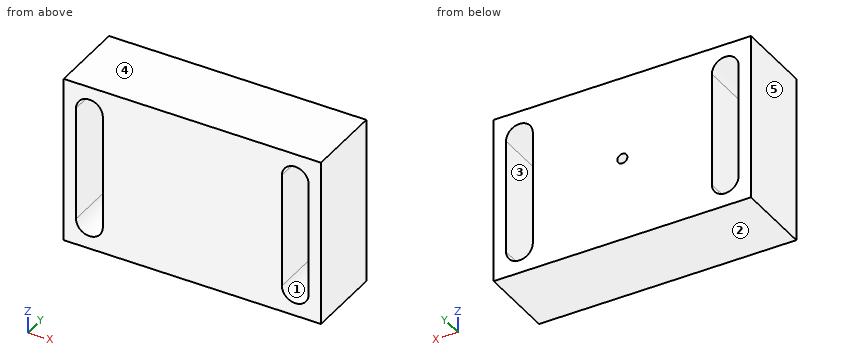
Autodesk Inventor part; units mm, degrees
ref_plane "YZ Plane" through (0, 0, 0) normal (1, 0, 0) x (0, 1, 0)
ref_plane "XZ Plane" through (0, 0, 0) normal (0, 1, 0) x (-1, 0, 0)
ref_plane "XY Plane" through (0, 0, 0) normal (0, 0, 1) x (1, 0, 0)
sketch "Sketch1" plane through (0, 0, 0) normal (0, 0, 1) x (1, 0, 0)
  line L0 (0, 0) -> (63.5, 0)
  line L1 (63.5, 0) -> (63.5, 19.05)
  line L2 (63.5, 19.05) -> (0, 19.05)
  line L3 (0, 19.05) -> (0, 0)
  dimension "d2" = 63.5
  dimension "d3" = 19.05
extrude "Extrusion1" add sketch "Sketch1" along normal blind 41.275
sketch "Sketch2" plane through (0, 19.05, 0) normal (0, 1, 0) x (1, 0, 0)
  line L0 (63.5, 0) -> (0, 0)
  line L1 (0, 0) -> (0, -41.275)
  point P0 (31.75, -20.6375)
  dimension "d4" = 20.6375
  dimension "d5" = 31.75
hole "Hole1" at (31.75, 19.05, 20.6375) direction (0, -1, 0) diameter 2.4638 depth 12.7 tip angle 118
sketch "Sketch3" plane through (0, 19.05, 0) normal (0, 1, 0) x (1, 0, 0)
  line L0 (6.35, -34.798) -> (6.35, -6.477) construction
  line L1 (3.048, -34.798) -> (3.048, -6.477)
  line L2 (9.652, -6.477) -> (9.652, -34.798)
  arc A0 (3.048, -34.798) -> (9.652, -34.798) centre (6.35, -34.798) ccw
  arc A1 (9.652, -6.477) -> (3.048, -6.477) centre (6.35, -6.477) ccw
  line L3 (0, 0) -> (0, -41.275)
  line L4 (63.5, -41.275) -> (0, -41.275)
  line L5 (63.5, 0) -> (0, 0)
  circle A2 centre (31.75, -20.6375) radius 1.2319
  circle A3 centre (31.75, -20.6375) radius 1.2319
  line L6 (31.75, -20.6375) -> (31.75, 0) construction
  line L7 (57.15, -34.798) -> (57.15, -6.477) construction
  line L8 (60.452, -34.798) -> (60.452, -6.477)
  line L9 (53.848, -6.477) -> (53.848, -34.798)
  arc A4 (53.848, -34.798) -> (60.452, -34.798) centre (57.15, -34.798) ccw
  arc A5 (60.452, -6.477) -> (53.848, -6.477) centre (57.15, -6.477) ccw
  point P0 (6.35, -20.6375)
  point P1 (57.15, -20.6375)
  dimension "d13" = 6.604
  dimension "d15" = 3.175
  dimension "d16" = 3.175
  dimension "d17" = 25.4
extrude "Extrusion2" cut sketch "Sketch3" against normal blind 25.4 contours L1 A1 L2 A0 | A4 L9 A5 L8
properties part number "Track Foot" material "Aluminum 6061"
For this review, take the finished solid that the model builds, in its own axes (mm). Face numbers are marked on the shaded views. A direction names the side the tool comes from. Round coordinates to 2 decimals unless told otherwise and drop trailing zeros. Write each loop counter-clockwise with the first axis right and the second up, starting at its lowest first coordinate (ties: lowest second). Pieces come first, ordered by that corner, then holes. Notation, with made-up numbers: (43.5, 0.25) -> (92.5, 0.25) arc R27 ccw to (92.5, 21.25) -> close; hole circle Ø5 at (-2.5, 27). An arc over 180 degrees is marked (long way). Use one line per item in the form item = value.
1) To check wall thickness, follow L1, parallel to X at y = 13.5, z = 35; L2, parallel to Z at x = 31.75, y = 12.25 (3 decimals). State the ranges of each line that lie inside material, in increasing order. Write a range as from..to.
Found:
L1 = 0..3.05, 9.65..53.85, 60.45..63.5
L2 = 0..19.406, 21.869..41.275
2) Take a section at A-A, the plane z = 11. Write out the cut boundary in (x, y).
Found:
outline = (0, 0) -> (3.05, 0) -> (3.05, 19.05) -> (0, 19.05) -> close; (9.65, 0) -> (53.85, 0) -> (53.85, 19.05) -> (9.65, 19.05) -> close; (60.45, 0) -> (63.5, 0) -> (63.5, 19.05) -> (60.45, 19.05) -> close
3) Take a section at D-D, the plane y = 3.75. Write out the cut boundary in (x, z) (3 decimals), and give its area (3 significant figures).
Found:
outline = (0, 0) -> (63.5, 0) -> (63.5, 41.275) -> (0, 41.275) -> close; hole (3.048, 6.477) arc R3.302 ccw to (9.652, 6.477) -> (9.652, 34.798) arc R3.302 ccw to (3.048, 34.798) -> close; hole (53.848, 6.477) arc R3.302 ccw to (60.452, 6.477) -> (60.452, 34.798) arc R3.302 ccw to (53.848, 34.798) -> close
area = 2,180 mm2
4) Clearance check with a flat-ended pin moving along its axis: pin 1 (6 mm diameter, centred on y = 16, z = 7, fed in from -X). State where the tip first meets the part, or that it passes through.
Found:
pin_1 = 0
5) Take a section at C-C, the plane x = 57.15. Write out the cut boundary in (y, z) (3 decimals).
Found:
outline = (0, 0) -> (19.05, 0) -> (19.05, 3.175) -> (0, 3.175) -> close; (0, 38.1) -> (19.05, 38.1) -> (19.05, 41.275) -> (0, 41.275) -> close
6) Tool access review of the marked faces 1 and 2: name each direction out of +Z, -Z, +X, -X, +Y, -Y from which nothing blocks a thin tool from reaching the whole face with its end or side.
Found:
face_1 = +Y, -Y
face_2 = -Z, +X, -X, +Y, -Y
7) Mouldability with a two-part tool opening along Z and no side actions: class the marked faces 3, 4 and 5 as +Z half, -Z half, draft (parallel to the pull), parting line (faces both ways), or undercut.
Found:
face_3 = undercut
face_4 = +Z half
face_5 = draft
8) Take a section at B-B, the plane y = 9.75. Count the separate pieces of the cut face and the enclosed holes in it, and give its area (3 significant figures).
Found:
separate_pieces = 1
enclosed_holes = 3
area = 2,170 mm2
